Model file for the job. Use its own axes, mm. A direction names the side the tool comes from. Round coordinates to 2 decimals unless told otherwise and drop trailing zeros. Order: outer loops, then holes, each group sorted by start corner. A loop starts at its lowest first (then second) coordinate and runs counter-clockwise, first axis right, second up. Notation, with made-up numbers: (85, 54) -> (131, 54) arc R23 cw to (131, 86) -> close; hole circle Ø1 at (48.25, 79). An arc over 180 degrees is marked (long way). Put each result on its own line as item: value. Start each with the question number.
Q1. Flat gauge pins, fed straight in: P1, Ø21.5, axis at x = -99, z = -45.5, coming from the -Y side; P2, Ø7, axis at x = -139, y = -11, coming from the -Z side; P3, Ø5, axis at x = -128, z = -65.5, coming from the -Y side. Where does each tip first touch, or does it go through?
Q2. Cut at C-C, the plane z = -8. List the corners of the cut face in (x, y).
Q3. 3-axis set-ups, long thin cutter, end or side, ignore diameter. For faces 5 (the face through (-68, -2.5, -4)), 6 (the face through (-114, -33, -36)), 7 (the face through (-129, -23, -3)), 8 (the face through (-138, -9, -17.5)): which of +Z, -Z, +X, -X, +Y, -Y reach the whole face in a straight line?
Q4. Pull direction X, two halves, no side cores. Call faces 1 (the face through (-129.07, -22.542, -62.546)), 2 (the face through (-134, -13, -9)), 3 (the face through (-69, -14, -34)), 4 (the face through (-130, -11, -43)): released by +X, released by -X, zero draft, split by the parting line, or undercut.
Q5. Cut at A-A, the plane y = -23. List the corners of the cut face in (x, z).
Q6. Probe L1, parallel to X at y = -16, z = -20; L2, parallel to X at y = -4, z = -4.5; L3, parallel to Y at x = -127.5, z = -8. List the from-to ranges inside material, lowest first.
Q7. Cut at D-D, the plane z = -36. List the corners of the cut face in (x, y).
Q8. Cut at B-B, the plane x = -83.5. List the corners of the cut face in (y, z).
from build123d import *

# Parameters (mm, degrees)
SKETCH5_W                  = 116
SKETCH5_H                  = 67
MAIN_BODY_DEPTH            = 14
SKETCH6_W                  = 116
SKETCH6_H                  = 67
SKETCH6_W_2                = 111
SKETCH6_H_2                = 62
RAIL_DEPTH                 = 2.5
SKETCH8_W                  = 134
SKETCH8_H                  = 4
COVER_DEPTH                = 72
SKETCH9_W                  = 14
SKETCH9_H                  = 14
SIPM_WINDOW_DEPTH          = 8
TUBE_ADAPTER_DEPTH         = 30
RIGHT_SCREW_TERMINAL_DEPTH = 10
RIGHT_SCREW_HOLE_REACH     = 136
SKETCH12_R                 = 1.524
LEFT_SCREW_TERMINAL_DEPTH  = 10
LEFT_SCREW_HOLE_REACH      = 136
SKETCH14_R                 = 1.524
SKETCH15_W                 = 37
SKETCH15_H                 = 18
SIPM_MOUNT_DEPTH           = 9
SKETCH17_W                 = 8.8
SKETCH17_H                 = 36
CUT_EXTRUDE1_DEPTH         = 16
ADAPTER_HOLE_REACH         = 146
SKETCH18_R                 = 1.524
SKETCH19_W                 = 116
SKETCH19_H                 = 11.5
CUT_EXTRUDE2_DEPTH         = 10


with BuildPart() as part:
    # Sketch5 → Main Body (new body)
    with BuildSketch(Plane(origin=(0, 0, 0), x_dir=(1, 0, 0), z_dir=(0, 1, 0))):
        Polygon((-124, 0), (-134, 0), (-134, 72), (0, 72), (0, 0), (-1.95326153, 0), align=None)
        with Locations((-68, 36)):
            Rectangle(SKETCH5_W, SKETCH5_H, mode=Mode.SUBTRACT)
    extrude(amount=-MAIN_BODY_DEPTH)

    # Sketch6 → Rail (add)
    with BuildSketch(Plane(origin=(0, 0, 0), x_dir=(1, 0, 0), z_dir=(0, 1, 0))):
        with Locations((-68, 36)):
            Rectangle(SKETCH6_W, SKETCH6_H)
        with Locations((-68, 36)):
            Rectangle(SKETCH6_W_2, SKETCH6_H_2, mode=Mode.SUBTRACT)
    extrude(amount=-RAIL_DEPTH)

    # Sketch8 → Cover (add)
    with BuildSketch(Plane.XY):
        with Locations((-67, -16)):
            Rectangle(SKETCH8_W, SKETCH8_H)
    extrude(amount=-COVER_DEPTH)

    # Sketch9 → SiPM Window (cut)
    with BuildSketch(Plane.ZY.offset(134)):
        with Locations((-36, -11)):
            Rectangle(SKETCH9_W, SKETCH9_H)
    extrude(amount=-SIPM_WINDOW_DEPTH, mode=Mode.SUBTRACT)

    # Sketch10 → Tube Adapter (add)
    with BuildSketch(Plane.XZ.offset(18)):
        with BuildLine():
            Line((-134, -13), (-134, -16))
            ThreePointArc((-134, -16), (-114, -36), (-134, -56))
            Line((-134, -56), (-134, -59))
            ThreePointArc((-134, -59), (-111, -36), (-134, -13))
        make_face()
    extrude(amount=TUBE_ADAPTER_DEPTH)

    # Sketch11 → Right Screw Terminal (add)
    with BuildSketch(Plane.XZ.offset(18)):
        with BuildLine():
            Line((-134, -59), (-134, -69))
            Line((-134, -69), (-124, -69))
            Line((-124, -69), (-124, -56.712315177))
            ThreePointArc((-124, -56.712315177), (-128.870830919, -58.420785547), (-134, -59))
        make_face()
    extrude(amount=RIGHT_SCREW_TERMINAL_DEPTH)

    # Sketch12 → Right Screw Hole (cut, up to next)
    with BuildSketch(Plane.ZY.offset(134), mode=Mode.PRIVATE) as right_screw_hole_sk1:
        with Locations((-64, -23)):
            Circle(SKETCH12_R)
    right_screw_hole_tool1 = extrude(right_screw_hole_sk1.sketch, amount=-RIGHT_SCREW_HOLE_REACH, mode=Mode.PRIVATE) & part.part
    add(right_screw_hole_tool1.solids().sort_by_distance((-134, -23, -64))[0], mode=Mode.SUBTRACT)

    # Sketch13 → Left Screw Terminal (add)
    with BuildSketch(Plane(origin=(0, -18, 0), x_dir=(-1, 0, 0), z_dir=(0, -1, 0))):
        with BuildLine():
            Line((134, 13), (134, 3))
            Line((134, 3), (124, 3))
            Line((124, 3), (124, 15.287684823))
            ThreePointArc((124, 15.287684823), (128.870830919, 13.579214453), (134, 13))
        make_face()
    extrude(amount=LEFT_SCREW_TERMINAL_DEPTH)

    # Sketch14 → Left Screw Hole (cut, up to next)
    with BuildSketch(Plane.ZY.offset(134), mode=Mode.PRIVATE) as left_screw_hole_sk1:
        with Locations((-8, -23)):
            Circle(SKETCH14_R)
    left_screw_hole_tool1 = extrude(left_screw_hole_sk1.sketch, amount=-LEFT_SCREW_HOLE_REACH, mode=Mode.PRIVATE) & part.part
    add(left_screw_hole_tool1.solids().sort_by_distance((-134, -23, -8))[0], mode=Mode.SUBTRACT)

    # Sketch15 → SiPM Mount (add)
    with BuildSketch(Plane.ZY.offset(134)):
        with Locations((-36, -9)):
            Rectangle(SKETCH15_W, SKETCH15_H)
    extrude(amount=SIPM_MOUNT_DEPTH)

    # Sketch17 → Cut-Extrude1 (cut)
    with BuildSketch(Plane.XZ.offset(18)):
        with Locations((-138.4, -36)):
            Rectangle(SKETCH17_W, SKETCH17_H)
    extrude(amount=-CUT_EXTRUDE1_DEPTH, mode=Mode.SUBTRACT)

    # Sketch18 → Adapter Hole (cut, up to next)
    with BuildSketch(Plane.ZY.offset(144), mode=Mode.PRIVATE) as adapter_hole_sk1:
        with Locations((-36, -40.5)):
            Circle(SKETCH18_R)
    adapter_hole_tool1 = extrude(adapter_hole_sk1.sketch, amount=-ADAPTER_HOLE_REACH, mode=Mode.PRIVATE) & part.part
    add(adapter_hole_tool1.solids().sort_by_distance((-144, -40.5, -36))[0], mode=Mode.SUBTRACT)

    # Sketch19 → Cut-Extrude2 (cut)
    with BuildSketch(Plane(origin=(0, 0, -2.5), x_dir=(-1, 0, 0), z_dir=(0, 0, -1))):
        with Locations((68, -8.25)):
            Rectangle(SKETCH19_W, SKETCH19_H)
    extrude(amount=-CUT_EXTRUDE2_DEPTH, mode=Mode.SUBTRACT)


solid = part.part
Ans:
1. P1: stops at y = -18
1. P2: stops at z = -54.5
1. P3: stops at y = -28
2. outline: (-134, -28) -> (-124, -28) -> (-124, -24.52) -> (-134, -24.52) -> close; (-134, -21.48) -> (-124, -21.48) -> (-124, -18) -> (0, -18) -> (0, 0) -> (-12.5, 0) -> (-12.5, -2.5) -> (-10, -2.5) -> (-10, -14) -> (-126, -14) -> (-126, -2.5) -> (-123.5, -2.5) -> (-123.5, 0) -> (-134, 0) -> close
3. face 5: +Z
3. face 6: -X, -Y
3. face 7: +Z, +X, -X, -Y
3. face 8: +Z, -X, +Y, -Y
4. face 1: zero draft
4. face 2: released by -X
4. face 3: undercut
4. face 4: undercut
5. outline: (-134, -69) -> (-124, -69) -> (-124, -65.52) -> (-134, -65.52) -> close; (-134, -62.48) -> (-124, -62.48) -> (-124, -56.71) arc R23 ccw to (-124, -15.29) -> (-124, -9.52) -> (-134, -9.52) -> (-134, -16) arc R20 cw to (-134, -56) -> close; (-134, -6.48) -> (-124, -6.48) -> (-124, -3) -> (-134, -3) -> close
6. L1: x = -143 to -142.8, -134 to 0
6. L2: x = -134 to -126, -10 to 0
6. L3: y = -28 to -24.52, -21.48 to 0
7. outline: (-143, -18) -> (-142.8, -18) -> (-142.8, -2) -> (-134, -2) -> (-134, -4) -> (-126, -4) -> (-126, -2.5) -> (-123.5, -2.5) -> (-123.5, 0) -> (-143, 0) -> close; (-126, -18) -> (-114, -18) -> (-114, -38.98) -> (-111, -38.98) -> (-111, -18) -> (0, -18) -> (0, 0) -> (-12.5, 0) -> (-12.5, -2.5) -> (-10, -2.5) -> (-10, -14) -> (-126, -14) -> close; (-114, -48) -> (-111, -48) -> (-111, -42.02) -> (-114, -42.02) -> close
8. outline: (-18, -72) -> (0, -72) -> (0, -67) -> (-2.5, -67) -> (-2.5, -69.5) -> (-14, -69.5) -> (-14, 0) -> (-18, 0) -> close; (-2.5, -5) -> (0, -5) -> (0, 0) -> (-2.5, 0) -> close
